Autodesk Inventor part; units mm, degrees
ref_plane "Start Plane" through (0, 0, -12.8489) normal (0, 0, 1) x (1, 0, 0)
ref_plane "End Plane" through (0, 0, 245.204) normal (0, 0, 1) x (1, 0, 0)
ref_plane "Work Plane4" through (-10, 0, 253.3619) normal (0.6321, 0, 0.7749) x (0.7749, 0, -0.6321)
ref_plane "Start Plane" through (0, 0, -12.8489) normal (0, 0, 1) x (1, 0, 0)
ref_plane "End Plane" through (0, 0, 245.204) normal (0, 0, 1) x (1, 0, 0)
sketch "Sketch" plane through (0, 0, 0) normal (0, 0, 1) x (1, 0, 0)
  line L0 (-10, -7) -> (-10, 7)
  line L1 (-7, 10) -> (7, 10)
  line L2 (10, 7) -> (10, -7)
  line L3 (7, -10) -> (-7, -10)
  arc A0 (-10, -7) -> (-7, -10) centre (-7, -7) ccw
  arc A1 (-7, 10) -> (-10, 7) centre (-7, 7) ccw
  arc A2 (10, 7) -> (7, 10) centre (7, 7) ccw
  arc A3 (7, -10) -> (10, -7) centre (7, -7) ccw
  arc A4 (-7, 8) -> (-8, 7) centre (-7, 7) ccw
  line L4 (-7, 8) -> (7, 8)
  arc A5 (8, 7) -> (7, 8) centre (7, 7) ccw
  line L5 (8, 7) -> (8, -7)
  arc A6 (7, -8) -> (8, -7) centre (7, -7) ccw
  line L6 (7, -8) -> (-7, -8)
  arc A7 (-8, -7) -> (-7, -8) centre (-7, -7) ccw
  line L7 (-8, -7) -> (-8, 7)
  line L8 (0, 14.8698) -> (0, -14.8698) construction
  line L9 (-14.8698, 0) -> (14.8698, 0) construction
  dimension "d7" = 3
  dimension "d10" = 20
  dimension "d11" = 20
  dimension "d12" = 2
  dimension "d15" = 10
  dimension "d16" = 10
extrude "Body" add sketch "Sketch" along normal up to surface (258.0529 mm away) from surface at -12.8489
sketch "Sketch3" plane through (0, 0, 0) normal (0, 0, 1) x (1, 0, 0)
  line L0 (0, 0) -> (10, 0)
ref_plane "Work Plane3" through (0, 0, 0) normal (0, -1, 0) x (1, 0, 0)
sketch "Sketch4" plane through (0, 0, 0) normal (0, -1, 0) x (1, 0, 0)
  line L0 (-2, -12.8489) -> (12, -12.8489)
  line L1 (-2, 245.204) -> (12, 245.204)
  dimension "d18" = 258.0529
ref_plane "Work Plane4" through (-10, 0, 253.3619) normal (0.6321, 0, 0.7749) x (0.7749, 0, -0.6321)
split "Split1" plane through (-10, 0, 253.3619) removes the side toward (0.6321, 0, 0.7749)
ref_plane "Work Plane5" through (10, 0, 257.4621) normal (-0.7749, 0, 0.6321) x (0.6321, 0, 0.7749)
split "Split2" plane through (10, 0, 257.4621) removes the side toward (-0.7749, 0, 0.6321)
ref_plane "Work Plane6" through (0, 10, -12.8489) normal (0, -0.7892, -0.6142) x (1, 0, 0)
split "Split3" plane through (0, 10, -12.8489) removes the side toward (0, -0.7892, -0.6142)
equation "\"d7\" = G_IR"
equation "\"d10\" = G_H"
equation "\"d11\" = G_W"
equation "\"d12\" = G_T"
equation "\"d15\" = 0.5 * d10"
equation "\"d16\" = 0.5 * d11"
equation "\"d3\" = G_L"
equation "\"G_W\" = 20"
equation "\"G_H\" = 20"
equation "\"G_T\" = 2"
equation "\"G_IR\" = 3"
equation "\"G_L\" = d18"
equation "\"G_OFFSET_START\" = 12.84887"
equation "\"G_OFFSET_END\" = 0"
equation "\"d13\" = -G_OFFSET_START"
equation "\"d14\" = G_OFFSET_END + B_L"
equation "\"B_L\" = 245.204"
properties part number "ISO 12633-2 - 20x20x2 - 258.05" material "Steel, Mild"
Design review of the part built by this model. Coordinates are the model's own, in mm. A direction names the side the tool comes from. Give positions to 0.01 mm unless a question says otherwise; leave off trailing zeros. Order: outer loops, then holes, each group sorted by start corner. A loop starts at its lowest first (then second) coordinate and runs counter-clockwise, first axis right, second up. Notation, with made-up numbers: M -8,44 L 10,44 A18 cw 10,64 Z; hole C 61,34.25 d8. An arc over 180 degrees is marked long. One line per question, with ' | ' between items. Start each with the question number.
Q1. The part is to be moulded in two halves that separate along Y. For faces 3 (the face through (8, 0, 113)), 4 (the face through (-10, 0, 110)), 5 (the face through (0, -10, 127)), say which applies: +Y half, -Y half, draft (parallel to the pull), parting line (faces both ways), or undercut.
Q2. We need section C-C (y = -1.75). Write out the cut boundary in (x, z), plus the area to 3 significant figures.
Q3. Machinability: for faces 1 (the face through (0, -8, 126)), 2 (the face through (10, 0, 112)), which of the approach directions +Z, -Z, +X, -X, +Y, -Y give a long, thin tool a straight path to every point of the face, cutting with its end or side? Answer none if there is none.
Q4. We need section A-A (z = 68.5). Write out the cut boundary in (x, y), plus the area to 3 significant figures.
Q5. We need section D-D (z = 6). Write out the cut boundary in (x, y), plus the area to 3 significant figures.
Q6. For L1, parallel to Y at x = -2.5, z = 217; L2, parallel to Z at x = -9, y = 4.25, list the stretches that pass through material, from the lowest coordinate up. Write a range as [from, to].
Q7. For pin 1 Ø6 at (x, y) = (3.5, -6.5) entering from +Z, flat-tipped, find the tip position at first contact; note if it passes through.
Q8. We need section B-B (x = 3.25). Write out the cut boundary in (y, z).
Returned:
1) face 3: undercut | face 4: draft | face 5: -Y half
2) outline: M -10,2.25 L -8,2.25 L -8,235.4 L -10,232.94 Z; M 8,2.25 L 10,2.25 L 10,237.05 L 8,238.68 Z | area: 935 mm2
3) face 1: +Z, -Z | face 2: +Z, -Z, +X, +Y, -Y
4) outline: M -10,-7 A3 ccw -7,-10 L 7,-10 A3 ccw 10,-7 L 10,7 A3 ccw 7,10 L -7,10 A3 ccw -10,7 Z; hole M -8,-7 A1 ccw -7,-8 L 7,-8 A1 ccw 8,-7 L 8,7 A1 ccw 7,8 L -7,8 A1 ccw -8,7 Z | area: 137 mm2
5) outline: M -10,-4.67 L -8,-4.67 L -8,7 A1 cw -7,8 L 7,8 A1 cw 8,7 L 8,-4.67 L 10,-4.67 L 10,7 A3 ccw 7,10 L -7,10 A3 ccw -10,7 Z | area: 87.2 mm2
6) L1: [-10, -8], [8, 10] | L2: [-5.46, 234.17]
7) pin 1: z = 244.47
8) outline: M -10,12.85 L -8,10.28 L -8,242.55 L -10,242.55 Z; M 8,-10.28 L 10,-12.85 L 10,242.55 L 8,242.55 Z
